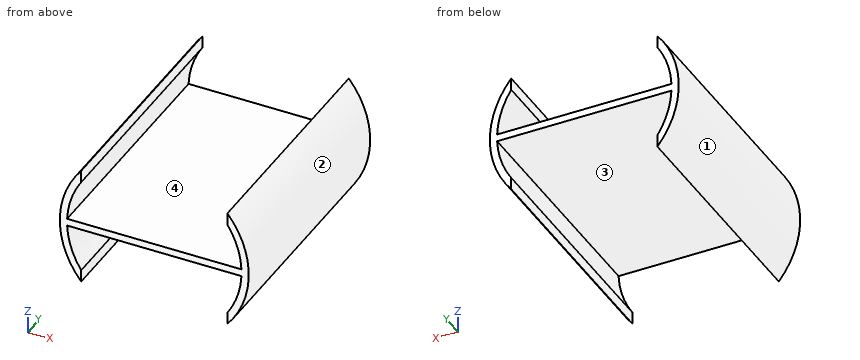
```python
from build123d import *

# Parameters (mm, degrees)
SKETCH2_R           = 25.85
BOSS_EXTRUDE1_DEPTH = 65
CUT_EXTRUDE1_START  = -100
CUT_EXTRUDE1_DEPTH  = 100


with BuildPart() as part:
    # Sketch2 → Boss-Extrude1 (new body)
    with BuildSketch(Plane(origin=(0, 0, 0), x_dir=(1, 0, 0), z_dir=(0, 1, 0))):
        with Locations(Location((0, 0, 0), (0, 0, 270))):
            Circle(SKETCH2_R)
    extrude(amount=BOSS_EXTRUDE1_DEPTH)

    # Sketch4 → Cut-Extrude1 (cut)
    with BuildSketch(Plane(origin=(0, 65, 0), x_dir=(1, 0, 0), z_dir=(0, 1, 0)).offset(CUT_EXTRUDE1_START)):
        with BuildLine():
            Line((-20, 16.377499809), (-20, 13.031596218))
            ThreePointArc((-20, 13.031596218), (0, 23.870955155), (20, 13.031596218))
            Line((20, 13.031596218), (20, 16.377499809))
            ThreePointArc((20, 16.377499809), (0, 25.85), (-20, 16.377499809))
        make_face()
        with BuildLine():
            ThreePointArc((20, 13.031596218), (0, 23.870955155), (-20, 13.031596218))
            Line((-20, 13.031596218), (-20, 11.370955155))
            Line((-20, 11.370955155), (20, 11.370955155))
            Line((20, 11.370955155), (20, 13.031596218))
        make_face()
        with BuildLine():
            ThreePointArc((-20, 13.031596218), (-22.735334875, 7.275097808), (-23.85, 1))
            Line((-23.85, 1), (23.85, 1))
            ThreePointArc((23.85, 1), (22.735334875, 7.275097808), (20, 13.031596218))
            Line((20, 13.031596218), (20, 11.370955155))
            Line((20, 11.370955155), (-20, 11.370955155))
            Line((-20, 11.370955155), (-20, 13.031596218))
        make_face()
        with BuildLine():
            ThreePointArc((-23.85, -1), (-22.735334875, -7.275097808), (-20, -13.031596218))
            Line((-20, -13.031596218), (-20, -11.370955155))
            Line((-20, -11.370955155), (20, -11.370955155))
            Line((20, -11.370955155), (20, -13.031596218))
            ThreePointArc((20, -13.031596218), (22.735334875, -7.275097808), (23.85, -1))
            Line((23.85, -1), (-23.85, -1))
        make_face()
        with BuildLine():
            Line((-20, -11.370955155), (-20, -13.031596218))
            ThreePointArc((-20, -13.031596218), (0, -23.870955155), (20, -13.031596218))
            Line((20, -13.031596218), (20, -11.370955155))
            Line((20, -11.370955155), (-20, -11.370955155))
        make_face()
        with BuildLine():
            Line((-20, -13.031596218), (-20, -16.377499809))
            ThreePointArc((-20, -16.377499809), (0, -25.85), (20, -16.377499809))
            Line((20, -16.377499809), (20, -13.031596218))
            ThreePointArc((20, -13.031596218), (0, -23.870955155), (-20, -13.031596218))
        make_face()
    extrude(amount=CUT_EXTRUDE1_DEPTH, mode=Mode.SUBTRACT)


solid = part.part
```
Verification items for the finished model (mm, model axes). Face numbers are marked on the shaded views. Round coordinates to 2 decimals unless told otherwise and drop trailing zeros. Write each loop counter-clockwise with the first axis right and the second up, starting at its lowest first coordinate (ties: lowest second). Pieces come first, ordered by that corner, then holes. Notation, with made-up numbers: (42, 45) -> (74, 45) arc R20 cw to (74, 74) -> close; hole circle Ø2 at (57, 24). An arc over 180 degrees is marked (long way). Write each question's results on one line, items separated by ' | '. Start each with the question number.
1. Material ranges on probe 1 along Z at (x, y) = (-17.5, 54.5); probe 2 along X at (y, z) = (11, 13.5); probe 3 along X at (y, z) = (23, 1.5), recorded low to high. Write a range as from..to.
2. Cross-section at C-C (x = -17). Enter the section's corners in (y, z).
3. Draft check along X on the marked faces 1, 2, 3 and 4. Enter one of: +X half, -X half, draft (parallel to the pull), parting line (faces both ways), or undercut.
4. Cross-section at D-D (z = 14). Enter the section's corners in (x, y).
5. Cross-section at A-A (z = -8). Enter the section's corners in (x, y), then the cut area to 3 significant figures.
6. Cross-section at B-B (y = 42.5). Enter the section's corners in (x, z).
7. Depth check by flat-ended pin: P1, Ø8, axis at x = 7.5, y = 37.5, coming from the -Z side; P2, Ø1.7, axis at y = 33, z = 15, coming from the +X side; P3, Ø8, axis at y = 31, z = -11.5, coming from the +X side; P4, Ø6, axis at x = -8, z = -3.5, coming from the +Y side. Enter the tip coordinate at first touch or a pass-through.
Solutions:
1) probe 1: z = -1..1 | probe 2: x = -22.04..-20, 20..22.04 | probe 3: x = -25.81..-23.82, 23.82..25.81
2) outline: (0, -1) -> (65, -1) -> (65, 1) -> (0, 1) -> close
3) face 1: -X half | face 2: +X half | face 3: undercut | face 4: undercut
4) outline: (-21.73, 0) -> (-20, 0) -> (-20, 65) -> (-21.73, 65) -> close; (20, 0) -> (21.73, 0) -> (21.73, 65) -> (20, 65) -> close
5) outline: (-24.58, 0) -> (-22.49, 0) -> (-22.49, 65) -> (-24.58, 65) -> close; (22.49, 0) -> (24.58, 0) -> (24.58, 65) -> (22.49, 65) -> close | area: 272 mm2
6) outline: (-23.85, -1) -> (23.85, -1) arc R23.87 cw to (20, -13.03) -> (20, -16.38) arc R25.85 ccw to (20, 16.38) -> (20, 13.03) arc R23.87 cw to (23.85, 1) -> (-23.85, 1) arc R23.87 cw to (-20, 13.03) -> (-20, 16.38) arc R25.85 ccw to (-20, -16.38) -> (-20, -13.03) arc R23.87 cw to start
7) P1: stops at z = -1 | P2: stops at x = 21.63 | P3: stops at x = 24.74 | P4: stops at y = 65
